Could you check a few things on this model? Use its own coordinates, in mm. Face numbers are marked on the shaded views. Give positions to 0.01 mm unless a question says otherwise; leave off trailing zeros. Order: outer loops, then holes, each group sorted by start corner. A loop starts at its lowest first (then second) coordinate and runs counter-clockwise, first axis right, second up. Notation, with made-up numbers: M 59,71 L 78,71 A4 cw 78,77 Z; hole C 31,33 d2. An arc over 180 degrees is marked long. Return JSON: item names as keys, results as strings. Group by question number.
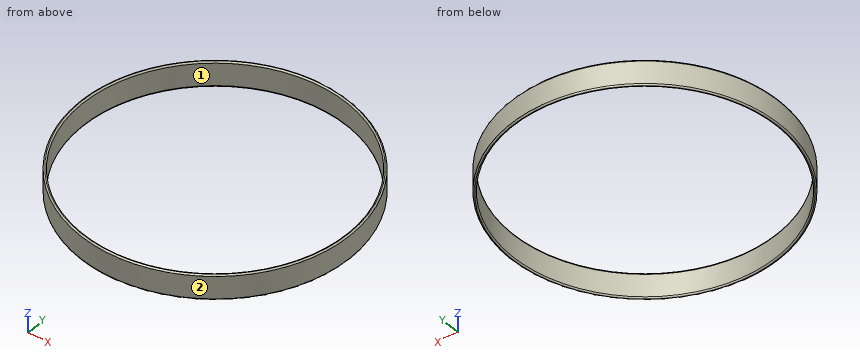
```python
from build123d import *

# Parameters (mm, degrees)
ESQUISSE1_R        = 50
BOSS_EXTRU_1_DEPTH = 9.35
COQUE1_T           = -1
CONG_1_R           = 0.5


with BuildPart() as part:
    # Esquisse1 → Boss.-Extru.1 (new body)
    with BuildSketch(Plane.XY):
        Circle(ESQUISSE1_R)
    extrude(amount=BOSS_EXTRU_1_DEPTH)

    # Coque1
    coque1_openings = [part.faces().sort_by_distance(p)[0] for p in [
        (0, 0, 9.35),
        (0, 0, 0),
    ]]
    offset(amount=COQUE1_T, openings=coque1_openings, kind=Kind.INTERSECTION)

    # Congé1
    cong_1_edges = [part.edges().sort_by_distance(p)[0] for p in [
        (-50, 0, 0),
        (-50, 0, 9.35),
        (-49, 0, 0),
        (-49, 0, 9.35),
    ]]
    fillet(cong_1_edges, radius=CONG_1_R - 0.0001)  # a hair under: the kernel refuses the full size


solid = part.part
```
1. I need wall thicknesses on L1, parallel to Y at x = 0, z = 6.5; L2, parallel to X at y = -38.5, z = 2.75; L3, parallel to X at y = -44.5, z = 7.5. Which ranges of each line are inside material? Lowest first, please. Write a range as from..to.
2. Imagine slicing it at C-C, the plane z = 6.25. Please give me the cut outline in (x, y).
3. If we mould it in two halves opening along Y, with no side actions, what happens to the marked faces 1 and 2? For each: pulls with the +Y half, pulls with the -Y half, needs draft (parallel to the pull), parting line crosses it, or undercut.
4. For pin 1 (1.5 mm diameter, centred on x = -17.5, z = 6, fed in from +Y); pin 2 (3 mm diameter, centred on x = 5.5, z = 1, fed in from -Y); pin 3 (2 mm diameter, centred on x = -21, z = 2, fed in from +Y); pin 4 (2 mm diameter, centred on x = 36.5, y = 28, fed in from -Z), each with a flat end and sliding along its axis, tell me the tip position at first contact or that it passes through.
Values:
{
 "1": {"L1": "y = -50..-49, 49..50", "L2": "x = -31.9..-30.31, 30.31..31.9", "L3": "x = -22.8..-20.51, 20.51..22.8"},
 "2": {"outline": "C 0,0 d100; hole C 0,0 d98"},
 "3": {"face 1": "undercut", "face 2": "parting line crosses it"},
 "4": {"pin 1": "stops at y = 47.11", "pin 2": "stops at y = -49.84", "pin 3": "stops at y = 45.83", "pin 4": "passes through"}
}
